Check sheet for the drawn part. Datum: minimum x, y, z corner. Units: mm. A direction names the side the tool comes from. Coordinates: 2 decimals unless noted, no trailing zeros. Loops run counter-clockwise (first coordinate to the right, second up) from the corner with the lowest first, then second, coordinate; pieces in that order, holes last.
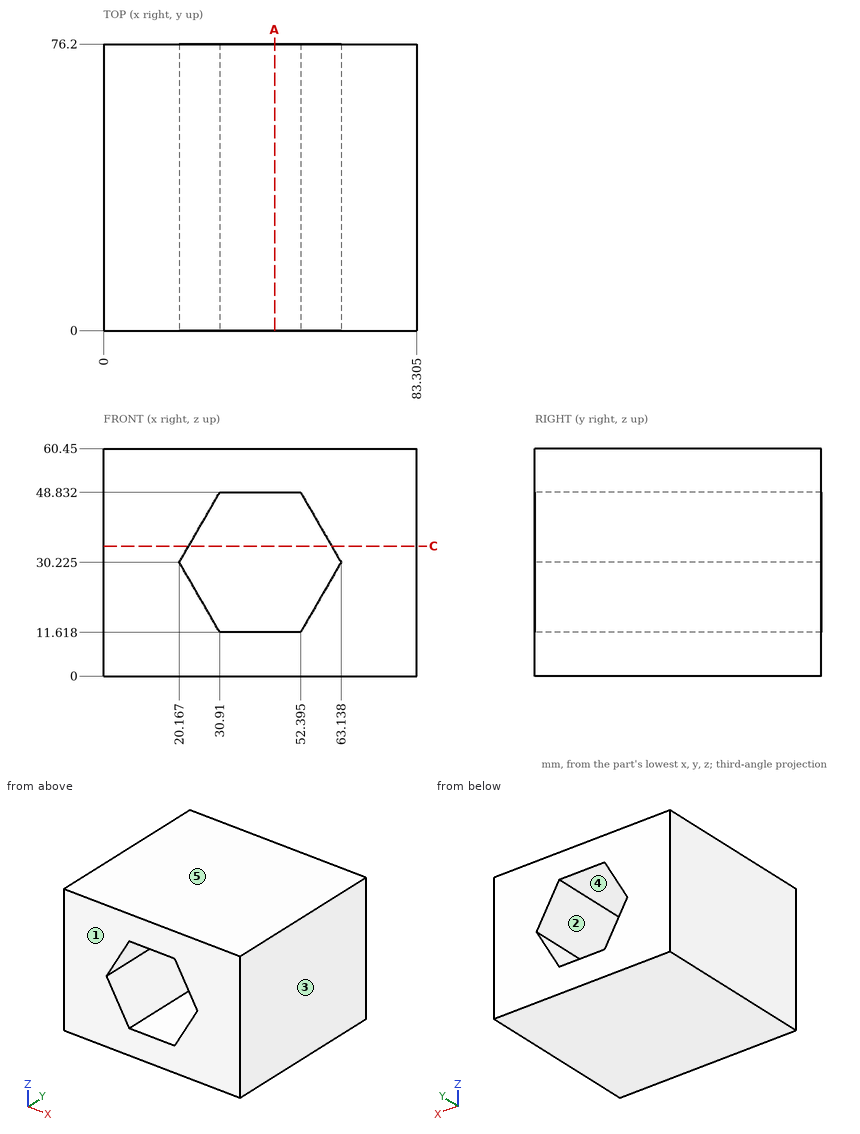
1) Section check C-C on z = 34.5. Enter the section's corners in (x, y) (1 decimal), plus the area to 3 significant figures.
Answer sheet:
outline: (0, 0) - (22.6, 0) - (22.6, 76.2) - (0, 76.2) - close; (60.7, 0) - (83.3, 0) - (83.3, 76.2) - (60.7, 76.2) - close
area: 3,450 mm2
2) Scan lines: line 1 (Z direction, x = 42.5, y = 70); line 2 (Z direction, x = 24.5, y = 65.5); line 3 (X direction, y = 40.5, z = 40.5) (1 decimal). Record each from-to range of solid material in increasing order.
Answer sheet:
line 1: z = 0 to 11.62, 48.83 to 60.45
line 2: z = 0 to 22.72, 37.73 to 60.45
line 3: x = 0 to 26.1, 57.2 to 83.3
3) Section check A-A on x = 45.5. Enter the section's corners in (y, z), plus the area to 3 significant figures.
Answer sheet:
outline: (0, 0) - (76.2, 0) - (76.2, 11.62) - (0, 11.62) - close; (0, 48.83) - (76.2, 48.83) - (76.2, 60.45) - (0, 60.45) - close
area: 1,770 mm2
4) Set-up check for the marked faces 1 and 2: record each of +Z, -Z, +X, -X, +Y, -Y from which the full face is reachable in a straight line by a thin tool's end or side.
Answer sheet:
face 1: +Z, -Z, +X, -X, -Y
face 2: +Y, -Y
5) Mould release check, pull along X, two halves, no side actions. Record for the marked faces 3, 4 and 5: +X half, -X half, draft (parallel to the pull), parting line (faces both ways), or undercut.
Answer sheet:
face 3: +X half
face 4: undercut
face 5: draft
